```python
from build123d import *

# Parameters (mm, degrees)
SKETCH1_R           = 1.75
BOSS_EXTRUDE1_DEPTH = 2.5
SKETCH2_W           = 40
SKETCH2_H           = 2.5
BOSS_EXTRUDE2_DEPTH = 100
FILLET1_R           = 5
CUT_EXTRUDE1_DEPTH  = 112.653481809


with BuildPart() as part:
    # Sketch1 → Boss-Extrude1 (new body)
    with BuildSketch(Plane(origin=(0, 0, 0), x_dir=(1, 0, 0), z_dir=(0, 1, 0))):
        with BuildLine():
            Line((20, 21), (-20, 21))
            Line((-20, 21), (-20, -16))
            ThreePointArc((-20, -16), (-18.535533906, -19.535533906), (-15, -21))
            Line((-15, -21), (15, -21))
            ThreePointArc((15, -21), (18.535533906, -19.535533906), (20, -16))
            Line((20, -16), (20, 21))
        make_face()
        with Locations(Location((14.75, -16, 0), (0, 0, 270))):
            Circle(SKETCH1_R, mode=Mode.SUBTRACT)
        with Locations(Location((-14.75, -16, 0), (0, 0, 90))):
            Circle(SKETCH1_R, mode=Mode.SUBTRACT)
    extrude(amount=BOSS_EXTRUDE1_DEPTH)

    # Sketch2 → Boss-Extrude2 (add)
    with BuildSketch(Plane(origin=(0, 2.5, 0), x_dir=(1, 0, 0), z_dir=(0, 1, 0))):
        with Locations((0, 19.75)):
            Rectangle(SKETCH2_W, SKETCH2_H)
    extrude(amount=BOSS_EXTRUDE2_DEPTH)

    # Fillet1
    fillet1_edges = [part.edges().sort_by_distance(p)[0] for p in [
        (-20, 102.5, -19.75),
        (20, 102.5, -19.75),
    ]]
    fillet(fillet1_edges, radius=FILLET1_R)

    # Sketch3 → Cut-Extrude1 (cut, through all)
    with BuildSketch(Plane.XY.offset(-18.5)):
        with BuildLine():
            Line((17.25, 92.632945603), (17.25, 39.235172541))
            ThreePointArc((17.25, 39.235172541), (16.957106781, 38.52806576), (16.25, 38.235172541))
            Line((16.25, 38.235172541), (14.75, 38.235172541))
            ThreePointArc((14.75, 38.235172541), (14.042893219, 38.52806576), (13.75, 39.235172541))
            Line((13.75, 39.235172541), (13.75, 97.556357651))
            ThreePointArc((13.75, 97.556357651), (14.042893219, 98.263464432), (14.75, 98.556357651))
            Line((14.75, 98.556357651), (16.25, 98.556357651))
            ThreePointArc((16.25, 98.556357651), (16.957106781, 98.263464432), (17.25, 97.556357651))
            Line((17.25, 97.556357651), (17.25, 92.632945603))
        make_face()
        with BuildLine():
            Line((-14.75, 38.235172541), (-16.25, 38.235172541))
            ThreePointArc((-16.25, 38.235172541), (-16.957106781, 38.52806576), (-17.25, 39.235172541))
            Line((-17.25, 39.235172541), (-17.25, 92.632945603))
            Line((-17.25, 92.632945603), (-17.25, 97.556357651))
            ThreePointArc((-17.25, 97.556357651), (-16.957106781, 98.263464432), (-16.25, 98.556357651))
            Line((-16.25, 98.556357651), (-14.75, 98.556357651))
            ThreePointArc((-14.75, 98.556357651), (-14.042893219, 98.263464432), (-13.75, 97.556357651))
            Line((-13.75, 97.556357651), (-13.75, 39.235172541))
            ThreePointArc((-13.75, 39.235172541), (-14.042893219, 38.52806576), (-14.75, 38.235172541))
        make_face()
    extrude(amount=-CUT_EXTRUDE1_DEPTH, mode=Mode.SUBTRACT)


solid = part.part
```
The listing builds one solid part. Answer for the finished solid, in the listing's coordinates (mm). A direction names the side the tool comes from. Round coordinates to 2 decimals unless told otherwise and drop trailing zeros. Loops run counter-clockwise (first coordinate to the right, second up) from the corner with the lowest first, then second, coordinate; pieces in that order, holes last.
1) A cutting plane is placed at D-D on z = 11. Determine the outline of the cut face in (x, y), plus the area to 3 significant figures.
Outcome:
outline: (-20, 0) - (20, 0) - (20, 2.5) - (-20, 2.5) - close
area: 100 mm2
2) A cutting plane is placed at A-A on y = 91.5. Determine the outline of the cut face in (x, z).
Outcome:
outline: (-20, -21) - (-17.25, -21) - (-17.25, -18.5) - (-20, -18.5) - close; (-13.75, -21) - (13.75, -21) - (13.75, -18.5) - (-13.75, -18.5) - close; (17.25, -21) - (20, -21) - (20, -18.5) - (17.25, -18.5) - close
3) For a pull along Y with two mould halves and no side action, classify faces 1 (the face through (-13.75, 69, -20)), 2 (the face through (0, 102.5, -20)), 3 (the face through (17.25, 69, -20)), 4 (the face through (-16.485, 1.232, 16.228)) as released by +Y, released by -Y, zero draft, split by the parting line, or undercut.
Outcome:
face 1: undercut
face 2: released by +Y
face 3: undercut
face 4: zero draft
4) Consider line 1 (X direction, y = 1.8, z = 16); line 2 (X direction, y = 63, z = -19); line 3 (Z direction, x = -14.75, y = 1.65). Determine where each line is inside the solid, lowest interval first.
Outcome:
line 1: x = -20 to -16.5, -13 to 13, 16.5 to 20
line 2: x = -20 to -17.25, -13.75 to 13.75, 17.25 to 20
line 3: z = -21 to 14.25, 17.75 to 21
5) For faces 5 (the face through (18, 1, 20)), 6 (the face through (0, 2.5, 1)), 7 (the face through (-17.25, 68, -20)), determine the directions among +Z, -Z, +X, -X, +Y, -Y from which every point of the face is accessible in a straight line to the end or side of a thin tool.
Outcome:
face 5: +Z, +X, +Y, -Y
face 6: +Z, +X, -X, +Y
face 7: +Z, -Z
6) A cutting plane is placed at C-C on y = 36. Determine the outline of the cut face in (x, z).
Outcome:
outline: (-20, -21) - (20, -21) - (20, -18.5) - (-20, -18.5) - close
7) Given P1, Ø1.2, axis at x = -15, z = -20, coming from the -Y side; P2, Ø8, axis at x = 1, y = 32.5, coming from the +Z side; P3, Ø5, axis at x = 12, z = -5.5, coming from the +Y side, each flat-ended and moving along its own axis, determine where each tip first touches the part or whether it passes through.
Outcome:
P1: stops at y = 0
P2: stops at z = -18.5
P3: stops at y = 2.5
8) A cutting plane is placed at B-B on x = 1.5. Determine the outline of the cut face in (y, z).
Outcome:
outline: (0, -21) - (102.5, -21) - (102.5, -18.5) - (2.5, -18.5) - (2.5, 21) - (0, 21) - close
